Answer from the drawing. Dimensions are ordinates in mm from the lowest x, y and z of the part. A direction names the side the tool comes from. Coordinates: 2 decimals unless noted, no trailing zeros. Write each loop counter-clockwise with the first axis right and the second up, starting at its lowest first coordinate (ties: lowest second). Pieces come first, ordered by that corner, then holes.
1) The part is cut by section B-B (x = 38). Determine the outline of the cut face in (y, z), then the cut area to 3 significant figures.
2) Each of these flat-tipped pins is pushed along its axis until it touches: pin 1 Ø16 at (x, z) = (35, 15) entering from +Y; pin 2 Ø10 at (x, y) = (44, 8.5) entering from -Z; pin 3 Ø10 at (y, z) = (34, 20) entering from +X. Where does it stop, or does it pass through?
3) Which of the six approach directions +Z, -Z, +X, -X, +Y, -Y give full straight-line access (tool end or side, diameter ignored) to the marked faces 4 and 5?
4) The part is cut by section A-A (z = 22). Determine the outline of the cut face in (x, y).
5) Determine the mould class of the marked faces 1, 2 and 3 for opening direction Z: +Z half, -Z half, draft (parallel to the pull), parting line (faces both ways), or undercut.
6) The part is cut by section D-D (z = 32.5). Determine the outline of the cut face in (x, y), then the cut area to 3 significant figures.
7) Find the intervals of material crossed by line 1 (Z direction, x = 30, y = 9); line 2 (X direction, y = 16.5, z = 20); line 3 (Y direction, x = 31, z = 38), in increasing order.
8) The part is cut by section C-C (y = 17). Determine the outline of the cut face in (x, z).
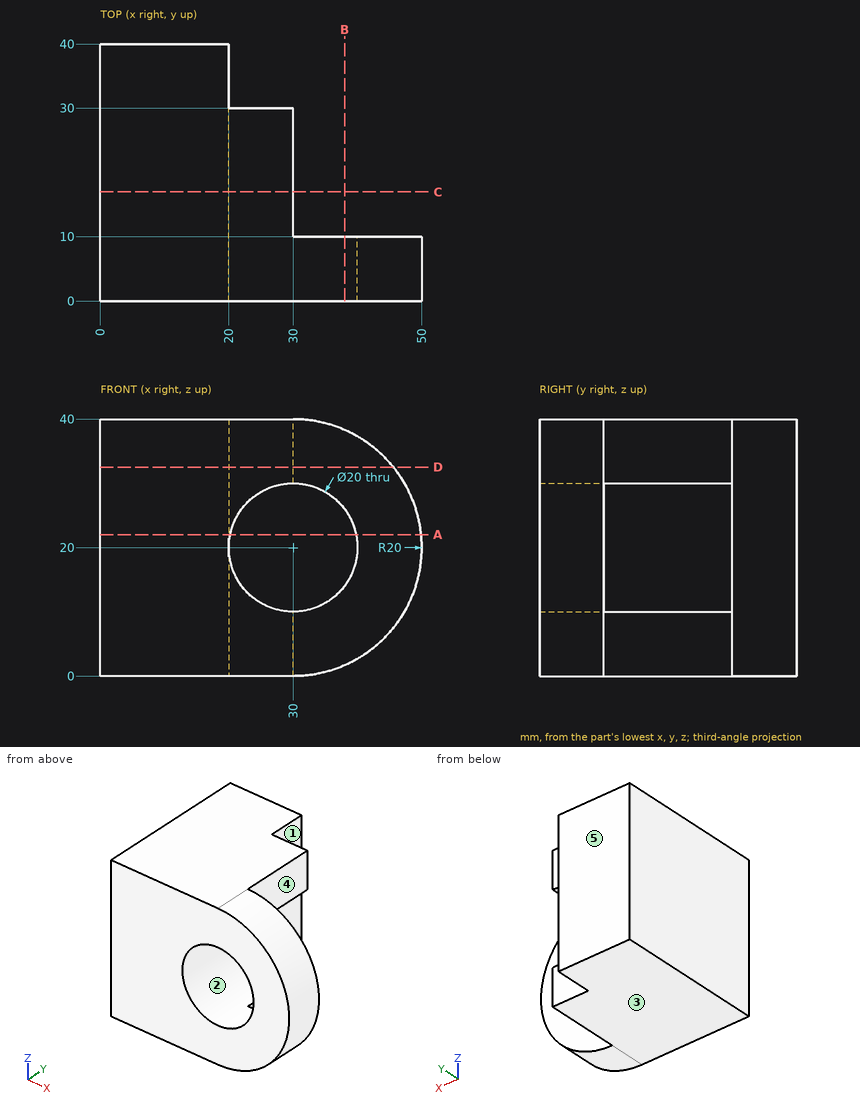
Reported:
1. outline: (0, 1.67) - (10, 1.67) - (10, 14) - (0, 14) - close; (0, 26) - (10, 26) - (10, 38.33) - (0, 38.33) - close
1. area: 247 mm2
2. pin 1: stops at y = 30
2. pin 2: stops at z = 2.14
2. pin 3: stops at x = 20.46
3. face 4: +Z, -Z, +X, +Y
3. face 5: +Z, -Z, +X, -X, +Y
4. outline: (0, 0) - (20.2, 0) - (20.2, 30) - (20, 30) - (20, 40) - (0, 40) - close; (39.8, 0) - (49.9, 0) - (49.9, 10) - (39.8, 10) - close
5. face 1: draft
5. face 2: undercut
5. face 3: -Z half
6. outline: (0, 0) - (45.61, 0) - (45.61, 10) - (30, 10) - (30, 30) - (20, 30) - (20, 40) - (0, 40) - close
6. area: 1,260 mm2
7. line 1: z = 0 to 10, 30 to 40
7. line 2: x = 0 to 20
7. line 3: y = 0 to 10
8. outline: (0, 0) - (30, 0) - (30, 10) arc R10 cw to (30, 30) - (30, 40) - (0, 40) - close
